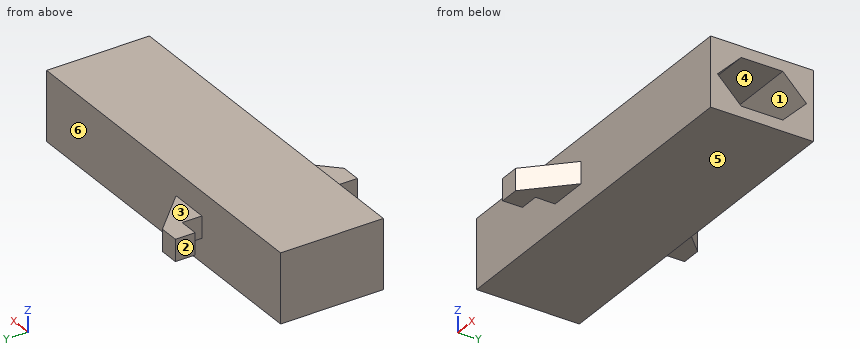
from build123d import *

# Parameters (mm, degrees)
F1_DEPTH  = 10
F2_W      = 21
F2_H      = 10
F3_DEPTH  = 9
F4_DEPTH  = 2
F5_DEPTH  = 3
F6_DEPTH  = 5
F7_DEPTH  = 2.5
F8_W      = 22.5
F8_H      = 12
F9_DEPTH  = 75
F11_DEPTH = 12
F12_SIZE  = 5.99999
F13_W     = 15
F13_H     = 5.5
F14_DEPTH = 10
F15_SIZE  = 9.99999
F16_W     = 5
F16_H     = 5.5
F17_DEPTH = 5
F18_W     = 15
F18_H     = 5.5
F19_DEPTH = 10
F20_SIZE  = 9.99999
F21_W     = 5
F21_H     = 5.5
F22_DEPTH = 5
F23_DEPTH = 5
F24_SIZE  = 5
F25_DEPTH = 5
F29_DEPTH = 25


# Not quite as in the source:
# - a fillet or chamfer is up to 0.001 mm smaller than in the source, because OpenCascade refuses the exact size
# - a feature of the source that left no trace in its solid (it failed there, or was rolled back) is left out


with BuildPart() as f1:
    # F0 (on Top) → F1 (new body)
    with BuildSketch(Plane.XY):
        Polygon((0, 10.5), (0, 0), (15, 0), align=None)
        Polygon((0, 10.5), (15, 0), (91, 0), (91, 21), (15, 21), align=None)
        Polygon((0, 21), (0, 10.5), (15, 21), align=None)
    extrude(amount=F1_DEPTH)

    # F2 (on face) → F3 (join)
    with BuildSketch(Plane(origin=(0, 0, 0), x_dir=(0, -1, 0), z_dir=(-1, 0, 0))):
        with Locations((-10.5, 5)):
            Rectangle(F2_W, F2_H)
    extrude(amount=F3_DEPTH)

    # F4 (add): a face of the model
    f4_faces = [f1.faces().sort_by_distance(p)[0] for p in [
        (41, 10.5, 10),
    ]]
    extrude(f4_faces, amount=F4_DEPTH)

    # F5 (add): a face of the model
    f5_faces = [f1.faces().sort_by_distance(p)[0] for p in [
        (41, 10.5, 12),
    ]]
    extrude(f5_faces, amount=F5_DEPTH)

    # F6 (add): a face of the model
    f6_faces = [f1.faces().sort_by_distance(p)[0] for p in [
        (41, 21, 7.5),
    ]]
    extrude(f6_faces, amount=F6_DEPTH)

    # F7 (add): a face of the model
    f7_faces = [f1.faces().sort_by_distance(p)[0] for p in [
        (41, 13, 15),
    ]]
    extrude(f7_faces, amount=F7_DEPTH)

    # F8 (on face) → F9 (cut)
    with BuildSketch(Plane.YZ.offset(91)):
        with Locations((13, 8.75)):
            Rectangle(F8_W, F8_H)
    extrude(amount=-F9_DEPTH, mode=Mode.SUBTRACT)

    # F10 (on face) → F11 (cut)
    with BuildSketch(Plane.XY.offset(2.75)):
        Polygon((16, 1.75), (16, 13), (1, 13), align=None)
        Polygon((1, 13), (16, 13), (16, 24.25), align=None)
    extrude(amount=F11_DEPTH, mode=Mode.SUBTRACT)

    # F12 (size 6 in the source; OpenCascade refuses exactly that, so slightly less here)
    f12_edges = [f1.edges().sort_by_distance(p)[0] for p in [
        (8.5, 7.375, 14.75),
        (8.5, 18.625, 14.75),
        (8.5, 7.375, 2.75),
        (8.5, 18.625, 2.75),
        (53.5, 1.75, 2.75),
        (53.5, 1.75, 14.75),
        (53.5, 24.25, 14.75),
        (53.5, 24.25, 2.75),
    ]]
    chamfer(f12_edges, length=F12_SIZE)

    # F13 (on face) → F14 (join)
    with BuildSketch(Plane(origin=(0, 26, 0), x_dir=(-1, 0, 0), z_dir=(0, 1, 0))):
        with Locations((-33.5, 8.75)):
            Rectangle(F13_W, F13_H)
    extrude(amount=F14_DEPTH)

    # F15 (size 10 in the source; OpenCascade refuses exactly that, so slightly less here)
    f15_edges = [f1.edges().sort_by_distance(p)[0] for p in [
        (41, 36, 8.75),
    ]]
    chamfer(f15_edges, length=F15_SIZE)

    # F16 (on face) → F17 (cut)
    with BuildSketch(Plane(origin=(26, 0, 0), x_dir=(0, -1, 0), z_dir=(-1, 0, 0))):
        with Locations((-28.5, 8.75)):
            Rectangle(F16_W, F16_H)
    extrude(amount=-F17_DEPTH, mode=Mode.SUBTRACT)

    # F18 (on face) → F19 (join)
    with BuildSketch(Plane.XZ):
        with Locations((33.5, 8.75)):
            Rectangle(F18_W, F18_H)
    extrude(amount=F19_DEPTH)

    # F20 (size 10 in the source; OpenCascade refuses exactly that, so slightly less here)
    f20_edges = [f1.edges().sort_by_distance(p)[0] for p in [
        (41, -10, 8.75),
    ]]
    chamfer(f20_edges, length=F20_SIZE)

    # F21 (on face) → F22 (cut)
    with BuildSketch(Plane(origin=(26, 0, 0), x_dir=(0, -1, 0), z_dir=(-1, 0, 0))):
        with Locations((2.5, 8.75)):
            Rectangle(F21_W, F21_H)
    extrude(amount=-F22_DEPTH, mode=Mode.SUBTRACT)

    # F23 (add): a face of the model
    f23_faces = [f1.faces().sort_by_distance(p)[0] for p in [
        (-9, 13, 8.75),
    ]]
    extrude(f23_faces, amount=F23_DEPTH)

    # F24
    f24_edges = [f1.edges().sort_by_distance(p)[0] for p in [
        (-14, 26, 8.75),
        (-14, 13, 17.5),
        (-14, 0, 8.75),
        (-14, 13, 0),
    ]]
    chamfer(f24_edges, length=F24_SIZE)

    # F25 (add): a face of the model
    f25_faces = [f1.faces().sort_by_distance(p)[0] for p in [
        (-14, 13, 8.75),
    ]]
    extrude(f25_faces, amount=F25_DEPTH)

    # F28 (on face) → F29 (cut)
    with BuildSketch(Plane.XY.offset(17.5)):
        Polygon((-36.3743491471, 0), (0.634705736, 0), (0.634705736, 13), (0.634705736, 34.4582907856), (-36.3743491471, 34.4582907856), align=None)
    extrude(amount=-F29_DEPTH, mode=Mode.SUBTRACT)


solid = f1.part
For this review, take the finished solid that the model builds, in its own axes (mm). Face numbers are marked on the shaded views. A direction names the side the tool comes from. Give positions to 0.01 mm unless a question says otherwise; leave off trailing zeros. Use CSV: the item, a comma, the result in double quotes.
Q1. To check wall thickness, follow probe 1 along Z at (x, y) = (62.5, 4.5); probe 2 along Y at (x, z) = (24.5, 12); probe 3 along Y at (x, z) = (58.5, 16.75). State the ranges of each line that lie inside material, in increasing order. Write a range as [from, to].
Conclusion:
probe 1,"[0, 6], [11.5, 17.5]"
probe 2,"[0, 5], [21, 26]"
probe 3,"[0, 26]"
Q2. For P1, Ø1.5, axis at y = 28, z = 7.5, coming from the -X side; P2, Ø1, axis at x = 17, z = 13, coming from the -Y side; P3, Ø8.5, axis at x = 67, y = 12, coming from the -Z side; P4, Ø5, axis at x = 34.5, y = -5, coming from the -Z side, all flat-tipped, find the tip position at first contact; note any pin that passes through.
Conclusion:
P1,"x = 31"
P2,"y = 0"
P3,"z = 0"
P4,"z = 6"
Q3. Tool access review of the marked faces 1, 2 and 3: name each direction out of +Z, -Z, +X, -X, +Y, -Y from which nothing blocks a thin tool from reaching the whole face with its end or side.
Conclusion:
face 1,"+X"
face 2,"+Z, -Z, -X, +Y"
face 3,"+Z, +X, -X, +Y"
Q4. Mouldability with a two-part tool opening along Z and no side actions: class the marked faces 4, 5 and 6 as pulls with the +Z half, pulls with the -Z half, needs draft (parallel to the pull), parting line crosses it, or undercut.
Conclusion:
face 4,"undercut"
face 5,"pulls with the -Z half"
face 6,"needs draft"
